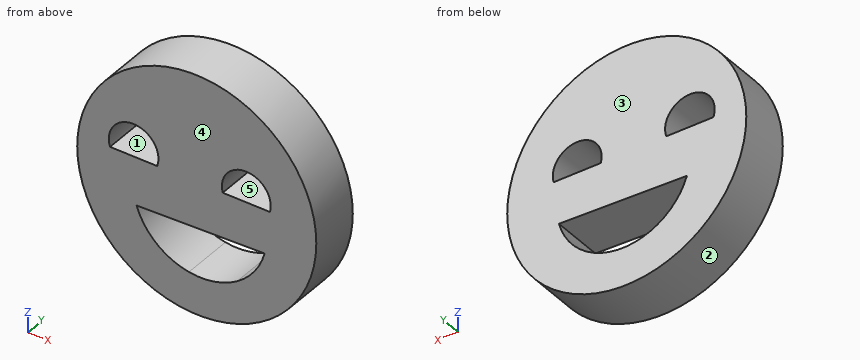
```python
from build123d import *

# Parameters (mm, degrees)
F0_R     = 58.853969
F1_DEPTH = 25.4


with BuildPart() as f1:
    # F0 (on Front) → F1 (new body)
    with BuildSketch(Plane.XZ):
        Circle(F0_R)
        with BuildLine():
            ThreePointArc((-3.849568, -39.504157), (-19.841394, -31.993164), (-29.622577, -17.279837))
            Line((-29.622577, -17.279837), (33.398006, -15.246916))
            ThreePointArc((33.398006, -15.246916), (28.39091, -26.088894), (19.836277, -34.421826))
            ThreePointArc((19.836277, -34.421826), (8.479387, -39.228113), (-3.849568, -39.504157))
        make_face(mode=Mode.SUBTRACT)
        with BuildLine():
            Line((-19.457968, 6.243975), (-42.691361, 6.243975))
            ThreePointArc((-42.691361, 6.243975), (-31.074665, 22.220387), (-19.457968, 6.243975))
        make_face(mode=Mode.SUBTRACT)
        with BuildLine():
            ThreePointArc((12.778366, 6.243975), (24.395064, 21.34293), (36.011763, 6.243975))
            Line((36.011763, 6.243975), (12.778366, 6.243975))
        make_face(mode=Mode.SUBTRACT)
    extrude(amount=F1_DEPTH)


solid = f1.part
```
Work out the finished part from the listing and answer in its coordinate system (mm). Face numbers are marked on the shaded views. A direction names the side the tool comes from. Round coordinates to 2 decimals unless told otherwise and drop trailing zeros. Write each loop counter-clockwise with the first axis right and the second up, starting at its lowest first coordinate (ties: lowest second). Pieces come first, ordered by that corner, then holes. Notation, with made-up numbers: (-15, -35.5) - (10, -35.5) arc R23 ccw to (10, -0.5) - close; hole circle Ø6 at (0.5, -30). An arc over 180 degrees is marked (long way). Return JSON: item names as keys, results as strings. Group by question number.
Q1. Each of these flat-tipped pins is pushed along its axis until it touches: pin 1 Ø11.5 at (x, y) = (-26.5, -16.5) entering from +Z; pin 2 Ø1 at (y, z) = (-4, 25.5) entering from +X; pin 3 Ø6 at (y, z) = (-3, -15) entering from +X. Where does it stop, or does it pass through?
Q2. Find the intervals of material crossed by L1, parallel to Z at x = -28, y = -5; L2, parallel to Z at x = 17, y = -6.75; L3, parallel to X at y = -3.5, z = -20.5, in increasing order.
Q3. The part is cut by section D-D on x = 32. Write down the section's boundary in (y, z), then the cut area to 3 significant figures.
Q4. The part is cut by section A-A on y = -10. Write down the section's boundary in (x, z).
Q5. The part is cut by section C-C on z = -24. Write down the section's boundary in (x, y), then the cut area to 3 significant figures.
Q6. The part is cut by section B-B on x = 0. Write down the section's boundary in (y, z), then the cut area to 3 significant figures.
Q7. For the marked faces 4 and 5, determine the directions among +Z, -Z, +X, -X, +Y, -Y from which every point of the face is accessible in a straight line to the end or side of a thin tool.
Q8. The mould has two halves that part along X. Classify the marked faces 1, 2 and 3: released by +X, released by -X, zero draft, split by the parting line, or undercut.
Solved:
{
 "1": {"pin 1": "z = 55.07", "pin 2": "x = 53.28", "pin 3": "x = 57.62"},
 "2": {"L1": "-51.77 to -21.33, -17.23 to 6.24, 21.83 to 51.77", "L2": "-56.35 to -36.12, -15.78 to 6.24, 18.8 to 56.35", "L3": "-55.17 to -28.39, 31.57 to 55.17"},
 "3": {"outline": "(-25.4, -49.39) - (0, -49.39) - (0, -19.5) - (-25.4, -19.5) - close; (-25.4, -15.29) - (0, -15.29) - (0, 6.24) - (-25.4, 6.24) - close; (-25.4, 18.63) - (0, 18.63) - (0, 49.39) - (-25.4, 49.39) - close", "area": "2,090 mm²"},
 "4": {"outline": "circle Ø117.71 at (0, 0); hole (-42.69, 6.24) - (-19.46, 6.24) arc R12.21 ccw (long way) to start; hole (-29.62, -17.28) arc R32.82 ccw to (-3.85, -39.5) arc R32.82 ccw to (19.84, -34.42) arc R32.82 ccw to (33.4, -15.25) - close; hole (12.78, 6.24) - (36.01, 6.24) arc R12.02 ccw (long way) to start"},
 "5": {"outline": "(-53.74, -25.4) - (-26.57, -25.4) - (-26.57, 0) - (-53.74, 0) - close; (29.75, -25.4) - (53.74, -25.4) - (53.74, 0) - (29.75, 0) - close", "area": "1,300 mm²"},
 "6": {"outline": "(-25.4, -58.85) - (0, -58.85) - (0, -39.92) - (-25.4, -39.92) - close; (-25.4, -16.32) - (0, -16.32) - (0, 58.85) - (-25.4, 58.85) - close", "area": "2,390 mm²"},
 "7": {"face 4": "+Z, -Z, +X, -X, -Y", "face 5": "+Y, -Y"},
 "8": {"face 1": "undercut", "face 2": "split by the parting line", "face 3": "zero draft"}
}
